CAD build for the part. Positions are in the model's coordinates, mm. Face numbers are marked on the shaded views. Give positions to 0.01 mm unless a question says otherwise; leave off trailing zeros. Loops run counter-clockwise (first coordinate to the right, second up) from the corner with the lowest first, then second, coordinate; pieces in that order, holes last. Notation, with made-up numbers: M 43.25,29.5 L 91.25,29.5 A17 ccw 91.25,34.5 Z; hole C 55.25,0.5 d11. An arc over 180 degrees is marked long. Answer as CSV lines item,"result".
```python
from build123d import *

# Parameters (mm, degrees)
SKETCH1_W           = 60
SKETCH1_H           = 30
BOSS_EXTRUDE3_DEPTH = 0.8
SKETCH4_W           = 0.8
SKETCH4_H           = 30
BOSS_EXTRUDE5_DEPTH = 30
SKETCH5_RX          = 15.076743355
SKETCH5_RY          = 15.045734075
BOSS_EXTRUDE6_DEPTH = 0.8
SKETCH6_R           = 5
SKETCH6_R_2         = 1.65
CUT_EXTRUDE2_DEPTH  = 10
SKETCH7_R           = 5
SKETCH7_R_2         = 1.65
CUT_EXTRUDE3_DEPTH  = 10


with BuildPart() as part:
    # Sketch1 → Boss-Extrude3 (new body)
    with BuildSketch(Plane(origin=(0, 0, 0), x_dir=(1, 0, 0), z_dir=(0, 1, 0))):
        with Locations((-9.504950495, -18.811881188)):
            Rectangle(SKETCH1_W, SKETCH1_H)
    extrude(amount=BOSS_EXTRUDE3_DEPTH)

    # Sketch4 → Boss-Extrude5 (add)
    with BuildSketch(Plane(origin=(0, 0, 0), x_dir=(-1, 0, 0), z_dir=(0, -1, 0))):
        with Locations((39.104950495, -18.811881188)):
            Rectangle(SKETCH4_W, SKETCH4_H)
    extrude(amount=BOSS_EXTRUDE5_DEPTH)

    # Sketch5 → Boss-Extrude6 (add)
    with BuildSketch(Plane(origin=(0, 0, 0), x_dir=(-1, 0, 0), z_dir=(0, -1, 0))):
        with Locations(Location((-20.627248494, -18.811881188), (0, 0, -73.484297411))):
            Ellipse(SKETCH5_RX, SKETCH5_RY)
    extrude(amount=-BOSS_EXTRUDE6_DEPTH)

    # Sketch6 → Cut-Extrude2 (cut)
    with BuildSketch(Plane(origin=(0, 0, 0), x_dir=(-1, 0, 0), z_dir=(0, -1, 0))):
        with Locations(Location((-21.694340642, -19.337305604, 0), (0, 0, 90))):
            Circle(SKETCH6_R)
        with Locations(Location((-21.694340642, -26.827036376, 0), (0, 0, 90))):
            Circle(SKETCH6_R_2)
        with Locations(Location((-29.349644864, -19.337305604, 0), (0, 0, 90))):
            Circle(SKETCH6_R_2)
        with Locations(Location((-21.694340642, -11.841250602, 0), (0, 0, 90))):
            Circle(SKETCH6_R_2)
        with Locations(Location((-14.079805527, -19.337305604, 0), (0, 0, 90))):
            Circle(SKETCH6_R_2)
        with Locations(Location((5.920194473, -19.337305604, 0), (0, 0, 90))):
            Circle(SKETCH6_R_2)
        with Locations(Location((25.920194473, -19.337305604, 0), (0, 0, 90))):
            Circle(SKETCH6_R_2)
        with Locations((-30.261708207, -582.328950324)):
            Circle(SKETCH6_R)
        with Locations((-37.91701243, -582.328950324)):
            Circle(SKETCH6_R_2)
        with Locations((-30.261708207, -574.832895322)):
            Circle(SKETCH6_R_2)
        with Locations((-22.647173092, -582.328950324)):
            Circle(SKETCH6_R_2)
        with Locations((-2.647173092, -582.328950324)):
            Circle(SKETCH6_R_2)
        with Locations((17.352826908, -582.328950324)):
            Circle(SKETCH6_R_2)
    extrude(amount=-CUT_EXTRUDE2_DEPTH, mode=Mode.SUBTRACT)

    # Mirror1: part across plane


with BuildPart() as part_1:
    add(part.part)
    add(part.part.mirror(Plane(origin=(0, -30, 0), x_dir=(0, 0, 1), z_dir=(0, -1, 0))))

    # Sketch7 → Cut-Extrude3 (cut)
    with BuildSketch(Plane(origin=(-38.704950495, 0, 0), x_dir=(0, 0, -1), z_dir=(1, 0, 0))):
        with Locations((-18.886165754, -29.145727498)):
            Circle(SKETCH7_R)
        with Locations((-18.928301582, -21.786074369)):
            Circle(SKETCH7_R_2)
        with Locations((-11.568184027, -29.145727498)):
            Circle(SKETCH7_R_2)
        with Locations((-18.886165754, -37.098993576)):
            Circle(SKETCH7_R_2)
        with Locations((-25.962216175, -29.145727498)):
            Circle(SKETCH7_R_2)
        with Locations((-18.928301582, -8.670402783)):
            Circle(SKETCH7_R_2)
        with Locations((-18.886165754, -48.835170272)):
            Circle(SKETCH7_R_2)
    extrude(amount=-CUT_EXTRUDE3_DEPTH, mode=Mode.SUBTRACT)


solid = part_1.part
```
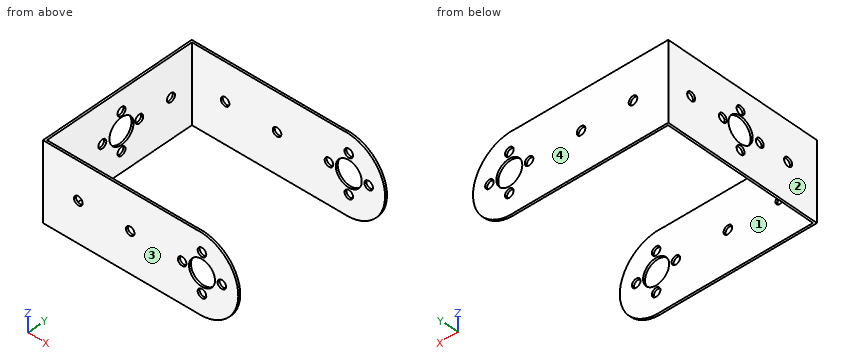
Q1. Pin check, flat tips, straight feed: P1, Ø3, axis at x = 21.69, z = 11.84, coming from the +Y side; P2, Ø5.5, axis at x = 14.08, z = 19.34, coming from the -Y side; P3, Ø10, axis at y = -7, z = 16, coming from the +X side. Stop position of each tip, or through.
Solution:
P1,"passes through"
P2,"stops at y = -60.8"
P3,"stops at x = -38.7"
Q2. Mould opens along Y. For the marked faces 1, 2, 3 and 4 say: released by +Y, released by -Y, zero draft, split by the parting line, or undercut.
Solution:
face 1,"undercut"
face 2,"zero draft"
face 3,"released by -Y"
face 4,"released by +Y"
Q3. Wall check: line 1 (Y direction, x = -31, z = 28.5); line 2 (X direction, y = -56, z = 32). Give the ranges that are in metal, low to high. Write a range as [from, to].
Solution:
line 1,"y = [-60.8, -60], [0, 0.8]"
line 2,"x = [-39.5, -38.7]"
Q4. Cut at B-B (x = 18). Write the cut outline in (y, z), and give its area (3 significant figures).
Solution:
outline,"M -60.8,3.81 L -60,3.81 L -60,15.97 L -60.8,15.97 Z; M -60.8,22.71 L -60,22.71 L -60,33.81 L -60.8,33.81 Z; M 0,3.81 L 0.8,3.81 L 0.8,15.97 L 0,15.97 Z; M 0,22.71 L 0.8,22.71 L 0.8,33.81 L 0,33.81 Z"
area,"37.2 mm²"
Q5. Cut at C-C (z = 16). Give the number of separate pieces and of enclosed holes in the cut face, and give its area (3 significant figures).
Solution:
separate pieces,"4"
enclosed holes,"0"
area,"149 mm²"
Q6. Cut at D-D (y = -40). Write the cut outline in (x, z), and give its area (3 significant figures).
Solution:
outline,"M -39.5,3.81 L -38.7,3.81 L -38.7,33.81 L -39.5,33.81 Z"
area,"24.0 mm²"
Q7. Cut at A-A (x = -2). Write the cut outline in (y, z), and give its area (3 significant figures).
Solution:
outline,"M -60.8,3.81 L -60,3.81 L -60,33.81 L -60.8,33.81 Z; M 0,3.81 L 0.8,3.81 L 0.8,33.81 L 0,33.81 Z"
area,"48.0 mm²"
